from build123d import *

# Parameters (mm, degrees)
SKETCH1_W           = 9
SKETCH1_H           = 1
SKETCH1_W_2         = 1
SKETCH1_H_2         = 9
BOSS_EXTRUDE1_DEPTH = 100


with BuildPart() as part:
    # Sketch1 → Boss-Extrude1 (new body)
    with BuildSketch(Plane(origin=(0, 0, 0), x_dir=(0, 0, -1), z_dir=(1, 0, 0))):
        with Locations((-15.137894846, 6.81112979)):
            Rectangle(SKETCH1_W, SKETCH1_H)
        with Locations((-10.137894846, 11.81112979)):
            Rectangle(SKETCH1_W_2, SKETCH1_H_2)
        with BuildLine():
            Line((-9.637894846, 7.31112979), (-10.637894846, 7.31112979))
            Line((-10.637894846, 7.31112979), (-10.637894846, 6.31112979))
            Line((-10.637894846, 6.31112979), (-10.137894846, 6.31112979))
            ThreePointArc((-10.137894846, 6.31112979), (-9.784341456, 6.4575764), (-9.637894846, 6.81112979))
            Line((-9.637894846, 6.81112979), (-9.637894846, 7.31112979))
        make_face()
    extrude(amount=BOSS_EXTRUDE1_DEPTH)


solid = part.part
Design review of the part built by this model. Coordinates are the model's own, in mm. A direction names the side the tool comes from. Round coordinates to 2 decimals unless told otherwise and drop trailing zeros. Write each loop counter-clockwise with the first axis right and the second up, starting at its lowest first coordinate (ties: lowest second). Pieces come first, ordered by that corner, then holes. Notation, with made-up numbers: (-12.75, 67) - (32.25, 67) arc R21 cw to (32.25, 87) - close; hole circle Ø10 at (82, -22.75). An arc over 180 degrees is marked (long way). Return JSON: item names as keys, results as strings. Group by question number.
Item 1: We need section B-B on z = 12.5. Write out the cut boundary in (x, y), and give its area (3 significant figures).
Item 2: We need section A-A on x = 40. Write out the cut boundary in (y, z).
Item 3: We need section C-C on y = 12.25. Write out the cut boundary in (x, z).
Item 4: For probe 1 along Z at (x, y) = (90, 12.25); probe 2 along Y at (x, z) = (75.5, 17.5), list the stretches that pass through material, from the lowest coordinate up. Write a range as [from, to].
Item 5: Machinability: for faces 1 (the face through (0, 7, 12)), 2 (the face through (49, 7.311, 15)), which of the approach directions +Z, -Z, +X, -X, +Y, -Y give a long, thin tool a straight path to every point of the face, cutting with its end or side? Answer none if there is none.
Item 6: Insertion check: P1, Ø2, axis at x = 29, z = 15.5, coming from the +Y side; P2, Ø2, axis at y = 9.5, z = 13.5, coming from the +X side. Each pin has a flat end and moves straight along its axis. Give the tip position at first contact, or say it passes through.
Model answer:
{
 "1": {"outline": "(0, 6.31) - (100, 6.31) - (100, 7.31) - (0, 7.31) - close", "area": "100 mm²"},
 "2": {"outline": "(6.31, 10.14) arc R0.5 ccw to (6.81, 9.64) - (16.31, 9.64) - (16.31, 10.64) - (7.31, 10.64) - (7.31, 19.64) - (6.31, 19.64) - close"},
 "3": {"outline": "(0, 9.64) - (100, 9.64) - (100, 10.64) - (0, 10.64) - close"},
 "4": {"probe 1": "z = [9.64, 10.64]", "probe 2": "y = [6.31, 7.31]"},
 "5": {"face 1": "+Z, -Z, -X, +Y, -Y", "face 2": "+Z, +X, -X, +Y"},
 "6": {"P1": "stops at y = 7.31", "P2": "passes through"}
}
